Could you check a few things on this model? Use its own coordinates, in mm. A direction names the side the tool comes from. Coordinates: 2 decimals unless noted, no trailing zeros. Order: outer loops, then holes, each group sorted by start corner. A loop starts at its lowest first (then second) coordinate and runs counter-clockwise, first axis right, second up. Notation, with made-up numbers: (-31, 80) - (-13, 80) arc R8 ccw to (-13, 86) - close; hole circle Ø3 at (67, 87.5). An arc over 180 degrees is marked (long way). Answer as a JSON object with one key per item and string values. Group by question number.
(1) We'd pull the mould along Y, two halves only. Please class faces 1 (the cylindrical face through (-27.15, -6.99, 2.03)), 2 (the flat face through (0, 0, 4)), 3 (the flat face through (-25, -2.9, 1)): pulls with the +Y half, pulls with the -Y half, needs draft (parallel to the pull), parting line crosses it, or undercut.
(2) Will these pins go through, and if not, where does the flat tip stop? P1, Ø3, axis at y = -5.5, z = -8, coming from the -X side; P2, Ø1.5, axis at x = -21, y = -2, coming from the -Z side; P3, Ø4.5, axis at x = -25, y = 0, coming from the -Z side.
(3) Imagine slicing it at C-C, the plane x = 21. Write out the boundary of the cut face in (y, z).
(4) Imagine slicing it at A-A, the plane x = -25. Write out the boundary of the cut face in (y, z).
(5) Please list where these lines run through material, in increasing order: probe 1 along X at (y, z) = (0.5, -4.5); probe 2 along Z at (x, y) = (11, 6.25); probe 3 along Z at (x, y) = (27, 1.25).
(6) Imagine slicing it at B-B, the plane z = -9.75. Write out the boundary of the cut face in (x, y), and give its area (3 significant figures).
(7) Which directions (+Z, -Z, +X, -X, +Y, -Y) give clear straight access to the entire face, cutting with the end or side of a thin tool? Please do faces 4 (the cylindrical face through (-6.386, -0.575, -8.168)), 5 (the flat face through (22.5, 1.47, 0.99)).
Autodesk Inventor part; units mm, degrees
ref_plane "YZ Plane" through (0, 0, 0) normal (1, 0, 0) x (0, 1, 0)
ref_plane "XZ Plane" through (0, 0, 0) normal (0, 1, 0) x (-1, 0, 0)
ref_plane "XY Plane" through (0, 0, 0) normal (0, 0, 1) x (1, 0, 0)
sketch "Sketch1" plane through (0, 0, 0) normal (0, 0, 1) x (1, 0, 0)
  line L0 (-30, -10) -> (30, -10)
  line L1 (30, -10) -> (30, 10)
  line L2 (30, 10) -> (-30, 10)
  line L3 (-30, 10) -> (-30, -10)
  line L4 (-30, -10) -> (30, 10) construction
  line L5 (30, -10) -> (-30, 10) construction
  circle A0 centre (0, 0) radius 9.9
  circle A1 centre (-25, 0) radius 1.65
  circle A2 centre (25, 0) radius 1.65
  line L6 (-25, 0) -> (25, 0) construction
  point P0 (-30, 0)
  dimension "d0" = 60
  dimension "d1" = 19.8
  dimension "d2" = 20
  dimension "d3" = 50
  dimension "d4" = 3.3
extrude "Extrusion1" add sketch "Sketch1" along normal blind 4 contours L3 L2 L1 L0 | A0
extrude "Extrusion2" add sketch "Sketch1" against normal blind 20 contours A0
fillet "Fillet1" radius 2 1 edges at (-9.9, 0, 0)
fillet "Fillet2" radius 10 4 edges at (30, 10, 2) (30, -10, 2) (-30, 10, 2) (-30, -10, 2)
sketch "Sketch2" plane through (0, 0, 0) normal (0, 0, -1) x (-1, 0, 0)
  arc A0 (-20, 10) -> (-20, -10) centre (-20, 0) ccw
  line L0 (-6.4506, -10) -> (-20, -10)
  arc A1 (-6.4506, 10) -> (-6.4506, -10) centre (0, 0) ccw
  line L1 (-20, 10) -> (-6.4506, 10)
  circle A2 centre (-25, 0) radius 1.65
  line L2 (25, 0) -> (-25, 0) construction
  line L3 (-23.3257, -2.9) -> (-26.6743, -2.9)
  line L4 (-26.6743, -2.9) -> (-28.3486, 0)
  line L5 (-28.3486, 0) -> (-26.6743, 2.9)
  line L6 (-26.6743, 2.9) -> (-23.3257, 2.9)
  line L7 (-23.3257, 2.9) -> (-21.6514, 0)
  line L8 (-21.6514, 0) -> (-23.3257, -2.9)
  circle A3 centre (25, 0) radius 1.65
  line L9 (23.3257, 2.9) -> (26.6743, 2.9)
  line L10 (26.6743, 2.9) -> (28.3486, 0)
  line L11 (28.3486, 0) -> (26.6743, -2.9)
  line L12 (26.6743, -2.9) -> (23.3257, -2.9)
  line L13 (23.3257, -2.9) -> (21.6514, 0)
  line L14 (21.6514, 0) -> (23.3257, 2.9)
  point P0 (25, 2.9)
  dimension "d11" = 5.8
  dimension "d12" = 5.8
extrude "Extrusion3" cut sketch "Sketch2" against normal blind 2 contours L3 L4 L5 L6 L7 L8 | L9 L10 L11 L12 L13 L14
sketch "Sketch3" plane through (0, 0, -20) normal (0, 0, -1) x (-1, 0, 0)
  circle A0 centre (0, 0) radius 9.9
  circle A1 centre (-5, 0) radius 1.5
  line L0 (0, 0) -> (0, 2.4769)
  circle A2 centre (5, 0) radius 1.5
  dimension "d15" = 3
  dimension "d16" = 10
extrude "Extrusion4" cut sketch "Sketch3" against normal through all contours A1 | A2
properties part number "GIRO_1" material "Steel, Mild, Welded"
Result set:
{
 "1": {"face 1": "pulls with the -Y half", "face 2": "needs draft", "face 3": "undercut"},
 "2": {"P1": "stops at x = -9.06", "P2": "stops at z = 0", "P3": "stops at z = 2"},
 "3": {"outline": "(-9.95, 0) - (9.95, 0) - (9.95, 4) - (-9.95, 4) - close"},
 "4": {"outline": "(-8.66, 0) - (-2.9, 0) - (-2.9, 2) - (-1.65, 2) - (-1.65, 4) - (-8.66, 4) - close; (1.65, 2) - (2.9, 2) - (2.9, 0) - (8.66, 0) - (8.66, 4) - (1.65, 4) - close"},
 "5": {"probe 1": "x = -9.89 to -6.41, -3.59 to 3.59, 6.41 to 9.89", "probe 2": "z = 0 to 4", "probe 3": "z = 2 to 4"},
 "6": {"outline": "circle Ø19.8 at (0, 0); hole circle Ø3 at (-5, 0); hole circle Ø3 at (5, 0)", "area": "294 mm^2"},
 "7": {"face 4": "+Z, -Z", "face 5": "-Z"}
}
